The listing builds one solid part. Answer for the finished solid, in the listing's coordinates (mm). Give positions to 0.01 mm unless a question says otherwise; leave off trailing zeros. Loops run counter-clockwise (first coordinate to the right, second up) from the corner with the lowest first, then second, coordinate; pieces in that order, holes last.
Item 1: Section C-C, the plane y = -514 is taken. Give the vertices of the cut face in (x, z).
Item 2: Section A-A, the plane x = -108.5 is taken. Give the vertices of the cut face in (y, z), and give its area (3 significant figures).
Item 3: Consider line 1 along Y through (x, z) = (96, 1.2); line 2 along X through (y, z) = (-723, 1.1); line 3 along Y through (x, z) = (67.5, 2.15). Determine where each line is inside the solid, lowest interval first.
Item 4: The mould has two halves that part along X. Classify faces 1 (the face through (74.423, -641.867, 2.535)), 2 (the face through (40, -711, 0)), 3 (the face through (-57.665, -710.377, 2.465)): pulls with the +X half, pulls with the -X half, needs draft (parallel to the pull), parting line crosses it, or undercut.
Item 5: This flat-tipped pin is pushed along its axis until it touches: pin 1 Ø1 at (y, z) = (-877.5, 0.5) entering from +X. Where does it stop, or does it pass through?
Item 6: Section B-B, the plane z = 2.95 is taken. Give the number of separate pieces and of enclosed holes in the cut face, and give its area (3 significant figures).
Autodesk Inventor part; units mm, degrees
ref_plane "YZ Plane" through (0, 0, 0) normal (1, 0, 0) x (0, 1, 0)
ref_plane "XZ Plane" through (0, 0, 0) normal (0, 1, 0) x (-1, 0, 0)
ref_plane "XY Plane" through (0, 0, 0) normal (0, 0, 1) x (1, 0, 0)
ref_plane "Work Plane1" through (0, 0, 0) normal (0, 0, 1) x (1, 0, 0)
sketch "Sketch1" plane through (0, 0, 0) normal (0, 0, 1) x (1, 0, 0)
  arc A0 (-157.6453, -1471.0012) -> (-157.6453, 28.9988) centre (-2920.1453, -721.0012) ccw
  line L0 (142.3547, 28.9988) -> (-157.6453, 28.9988)
  arc A1 (142.3547, -1471.0012) -> (142.3547, 28.9988) centre (-2620.1453, -721.0012) ccw
  line L1 (142.3547, -1471.0012) -> (-157.6453, -1471.0012)
  point P0 (0, 0)
extrude "Extrusion1" add sketch "Sketch1" along normal blind 5
sketch "Sketch2" plane through (0, 0, 5) normal (0, 0, 1) x (1, 0, 0)
  circle A0 centre (-136.8008, 12.9988) radius 3.1
  circle A1 centre (-132.5804, -3.0012) radius 3.1
  circle A2 centre (-83.4222, 12.9988) radius 3.1
  circle A3 centre (-79.2018, -3.0012) radius 3.1
  circle A4 centre (-30.0436, 12.9988) radius 3.1
  circle A5 centre (-25.8232, -3.0012) radius 3.1
  circle A6 centre (23.335, 12.9988) radius 3.1
  circle A7 centre (27.5554, -3.0012) radius 3.1
  circle A8 centre (76.7136, 12.9988) radius 3.1
  circle A9 centre (80.934, -3.0012) radius 3.1
  circle A10 centre (130.0922, 12.9988) radius 3.1
  circle A11 centre (134.3126, -3.0012) radius 3.1
  circle A12 centre (-132.5804, -1439.0012) radius 3.1
  circle A13 centre (-136.8008, -1455.0012) radius 3.1
  circle A14 centre (-79.2018, -1439.0012) radius 3.1
  circle A15 centre (-83.4222, -1455.0012) radius 3.1
  circle A16 centre (-25.8232, -1439.0012) radius 3.1
  circle A17 centre (-30.0436, -1455.0012) radius 3.1
  circle A18 centre (27.5554, -1439.0012) radius 3.1
  circle A19 centre (23.335, -1455.0012) radius 3.1
  circle A20 centre (80.934, -1439.0012) radius 3.1
  circle A21 centre (76.7136, -1455.0012) radius 3.1
  circle A22 centre (134.3126, -1439.0012) radius 3.1
  circle A23 centre (130.0922, -1455.0012) radius 3.1
  point P0 (0, 0)
extrude "Extrusion2" cut sketch "Sketch2" against normal blind 5
sketch "Sketch3" plane through (0, 0, 5) normal (0, 0, 1) x (1, 0, 0)
  arc A0 (-61.0788, -861.1613) -> (-61.0788, -580.841) centre (-7.6453, -721.0012) ccw construction
  arc A1 (-60.5809, -850.6076) -> (-60.5809, -591.3948) centre (-7.6453, -721.0012) ccw construction
  circle A2 centre (62.3547, -842.2447) radius 50
  circle A3 centre (132.3547, -721.0012) radius 40
  circle A4 centre (80.9262, -612.5802) radius 30
  circle A5 centre (-13.2241, -710.6475) radius 85.0368
  line L0 (45.6684, -649.3048) -> (60.1495, -634.2212) construction
  line L1 (71.5984, -716.6801) -> (92.4555, -718.1635) construction
  line L2 (132.3547, -721.0012) -> (62.3547, -842.2447) construction
  line L3 (132.3547, -721.0012) -> (80.9262, -612.5802) construction
  line L4 (93.7833, -639.6855) -> (115.2119, -684.8609) construction
  line L5 (112.3547, -755.6422) -> (87.3547, -798.9435) construction
  line L6 (62.3547, -842.2447) -> (-60.5809, -850.6076) construction
  arc A6 (-157.6453, -1471.0012) -> (-157.6453, 28.9988) centre (-2920.1453, -721.0012) ccw construction
  point P0 (0, 0)
  dimension "d9" = 100
  dimension "d8" = 10
  dimension "d10" = 80
  dimension "d11" = 60
  dimension "d12" = 50
extrude "Extrusion3" cut sketch "Sketch3" against normal through all contours A2 | A3 | A4
properties part number "Top_Blade"
Worked answers:
1. outline: (-65.14, 0) - (234.86, 0) - (234.86, 5) - (-65.14, 5) - close
2. outline: (-1471, 0) - (-1258.18, 0) - (-1258.18, 5) - (-1471, 5) - close; (-183.83, 0) - (29, 0) - (29, 5) - (-183.83, 5) - close
2. area: 2,130 mm2
3. line 1: y = -1471 to -879.23, -805.26 to -737.68, -704.32 to -638.52, -586.64 to 29
3. line 2: x = -57.65 to 92.4, 172.3 to 242.35
3. line 3: y = -1471 to -891.98, -792.51 to -639.41, -585.75 to 29
4. face 1: undercut
4. face 2: needs draft
4. face 3: pulls with the -X half
5. pin 1: stops at x = 238.1
6. separate pieces: 1
6. enclosed holes: 27
6. area: 434,000 mm2
